```python
from build123d import *

# Parameters (mm, degrees)
SKETCH_W          = 355
SKETCH_H          = 80
PAD_DEPTH         = 15
SKETCH001_W       = 6.5
SKETCH001_H       = 6
POCKET_DEPTH      = 177.501
POCKET_DEPTH_BACK = -177.501


with BuildPart() as part:
    # Sketch → Pad (new body)
    with BuildSketch(Plane.XY):
        Rectangle(SKETCH_W, SKETCH_H)
    extrude(amount=PAD_DEPTH)

    # Sketch001 → Pocket (cut, two sides)
    with BuildSketch(Plane.YZ) as pocket_sk:
        with Locations((-30.75, 12)):
            Rectangle(SKETCH001_W, SKETCH001_H)
    extrude(amount=-POCKET_DEPTH, mode=Mode.SUBTRACT)
    extrude(pocket_sk.sketch, amount=-POCKET_DEPTH_BACK, mode=Mode.SUBTRACT)


solid = part.part
```
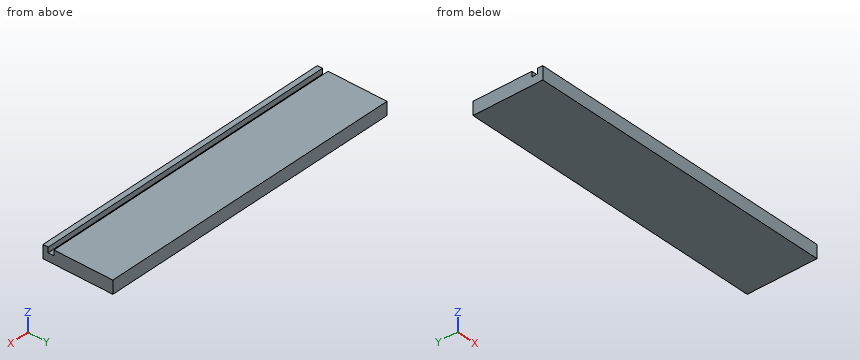
Design review of the part built by this model. Coordinates are the model's own, in mm. Coordinates: 2 decimals unless noted, no trailing zeros. Order: outer loops, then holes, each group sorted by start corner. A loop starts at its lowest first (then second) coordinate and runs counter-clockwise, first axis right, second up. Notation, with made-up numbers: (31, 66) - (80, 66) arc R14 cw to (80, 88) - close; hole circle Ø11 at (52, 65). An arc over 180 degrees is marked (long way). Answer in a Markdown table with one row per item.
(1) Consider section B-B on x = -83. State the section outline as (y, z) points.
Checked values:
| item | result |
|---|---|
| outline | (-40, 0) - (40, 0) - (40, 15) - (-27.5, 15) - (-27.5, 9) - (-34, 9) - (-34, 15) - (-40, 15) - close |
(2) Clearance check with a flat-ended pin moving along its axis: pin 1 (3 mm diameter, centred on x = 72.5, y = -31, fed in from +Z). State where the tip first meets the part, or that it passes through.
Checked values:
| item | result |
|---|---|
| pin 1 | z = 9 |
(3) Consider section A-A on z = 11.5. State the section outline as (x, y) points, plus the area to 3 significant figures.
Checked values:
| item | result |
|---|---|
| outline | (-177.5, -40) - (177.5, -40) - (177.5, -34) - (-177.5, -34) - close; (-177.5, -27.5) - (177.5, -27.5) - (177.5, 40) - (-177.5, 40) - close |
| area | 26,100 mm^2 |
(4) Wall thickness on line 1 along Y through (x, z) = (138.5, 11.75): over which ranges is the line inside the solid? List them lowest first. Write a range as from..to.
Checked values:
| item | result |
|---|---|
| line 1 | -40..-34, -27.5..40 |
